Build history of the part. All positions in model axes, mm. A direction names the side the tool comes from. Round coordinates to 2 decimals unless told otherwise and drop trailing zeros. Write item = value, one per line.
from build123d import *

# Parameters (mm, degrees)
SKETCH1_W               = 25.4
SKETCH1_H               = 82.55
BOSS_EXTRUDE1_DEPTH     = 6.35
SKETCH2_R               = 1.5875
CUT_EXTRUDE1_DEPTH      = 44.649033494
SKETCH3_W               = 19.05
SKETCH3_H               = 60.325
CUT_EXTRUDE2_DEPTH      = 1.5875
CUT_EXTRUDE3_DEPTH      = 44.649033494
CUT_EXTRUDE3_DEPTH_BACK = 44.649033494
SKETCH5_W               = 9.525
SKETCH5_H               = 6.35
BOSS_EXTRUDE2_DEPTH     = 6.35


with BuildPart() as part:
    # Sketch1 → Boss-Extrude1 (new body)
    with BuildSketch(Plane.XY):
        Rectangle(SKETCH1_W, SKETCH1_H)
    extrude(amount=BOSS_EXTRUDE1_DEPTH)

    # Sketch2 → Cut-Extrude1 (cut, through all)
    with BuildSketch(Plane.XY.offset(6.35)):
        with Locations((-6.35, 15.875)):
            Circle(SKETCH2_R)
        with Locations(Location((6.35, 15.875, 0), (0, 0, 180))):
            Circle(SKETCH2_R)
    extrude(amount=-CUT_EXTRUDE1_DEPTH, mode=Mode.SUBTRACT)

    # Sketch3 → Cut-Extrude2 (cut)
    with BuildSketch(Plane.XY.offset(6.35)):
        with Locations((0, -11.1125)):
            Rectangle(SKETCH3_W, SKETCH3_H)
    extrude(amount=-CUT_EXTRUDE2_DEPTH, mode=Mode.SUBTRACT)

    # Sketch5 → Cut-Extrude3 (cut, two sides: drawn at the far end of the back side and taken through both)
    with BuildSketch(Plane.XY.offset(6.35).offset(-CUT_EXTRUDE3_DEPTH_BACK)):
        with Locations((0, 35.56)):
            Rectangle(SKETCH5_W, SKETCH5_H)
    extrude(amount=CUT_EXTRUDE3_DEPTH + CUT_EXTRUDE3_DEPTH_BACK, mode=Mode.SUBTRACT)

    # Sketch6 → Boss-Extrude2 (add)
    with BuildSketch(Plane.XY.offset(6.35)):
        Polygon((-7.3025, 41.275), (7.3025, 41.275), (7.3025, 19.05), (4.7625, 19.05), (4.7625, 38.735), (-4.7625, 38.735), (-4.7625, 19.05), (-7.3025, 19.05), align=None)
    extrude(amount=BOSS_EXTRUDE2_DEPTH)


solid = part.part
1. Tool access for faces 4 (the face through (4.762, 31, 8)), 5 (the face through (0, 32.385, 3)), 6 (the face through (0, -11, 4.762)), 7 (the face through (-7.302, 30, 9)): list every direction of +Z, -Z, +X, -X, +Y, -Y with a clear straight run to the whole face (end or side of a thin tool).
Responses:
face_4 = +Z
face_5 = +Z, -Z
face_6 = +Z, -Y
face_7 = +Z, -X, +Y, -Y
2. Band-saw the part on C-C (z = 3). Count the separate pieces of the cut face and the enclosed holes in it, plus the area to 3 significant figures.
Responses:
separate_pieces = 1
enclosed_holes = 3
area = 2,020 mm²
3. Probe probe 1 along Y at (x, z) = (6.35, 1.95) (1 decimal); probe 2 along Y at (x, z) = (3.5, 5.25) (3 decimals); probe 3 along X at (y, z) = (21, 11.5). List the from-to ranges inside material, lowest first.
Responses:
probe_1 = -41.3 to 14.3, 17.5 to 41.3
probe_2 = 19.05 to 32.385, 38.735 to 41.275
probe_3 = -7.3 to -4.76, 4.76 to 7.3
4. Mould opens along X. For faces 1 (the face through (9.525, -12, 6)), 2 (the face through (0, 1, 0)), 3 (the face through (-12.7, -1, 3)) say: pulls with the +X half, pulls with the -X half, needs draft (parallel to the pull), parting line crosses it, or undercut.
Responses:
face_1 = undercut
face_2 = needs draft
face_3 = pulls with the -X half
5. Flat gauge pins, fed straight in: pin 1 (4.5 mm diameter, centred on x = -10, y = 3.5, fed in from +Z); pin 2 (1.9 mm diameter, centred on y = 32.5, z = 9, fed in from +X); pin 3 (4 mm diameter, centred on x = 4, z = 7, fed in from -Y). Where does each tip first touch, or does it go through?
Responses:
pin_1 = 6.35
pin_2 = 7.3
pin_3 = 19.05
